Read the model definition and answer for the solid it produces. Units are mm, in the model's axes. A direction names the side the tool comes from. Coordinates: 2 decimals unless noted, no trailing zeros. Order: outer loops, then holes, each group sorted by start corner. A loop starts at its lowest first (then second) coordinate and runs counter-clockwise, first axis right, second up. Notation, with made-up numbers: M 34,-38.75 L 59,-38.75 A17 cw 59,-14.75 Z; hole C 16.5,36.25 d9. An arc over 180 degrees is marked long. One line per question, with ' | ' between items. Start each with the question number.
1) A tool of negligible diameter and unlimited length cuts with its end or side. For faces 1 (the face through (7, -7, 0)), 2 (the face through (-7.559, -5.796, 36.51)), from which of +Z, -Z, +X, -X, +Y, -Y can it reach the whole face along a straight path? Write none if from no direction.
2) Consider probe 1 along X at (y, z) = (7, 51.5); probe 2 along X at (y, z) = (8.5, 41); probe 3 along Y at (x, z) = (2, 38.5). Determine where each line is inside the solid, lowest interval first.
3) Find section A-A, the plane z = 38. Count the separate pieces of the cut face and the enclosed holes in it, plus the area to 3 significant figures.
4) The mould has two halves that part along Y. Classify faces 3 (the face through (-6.883, -30.995, 35.496)), 4 (the face through (-2, 8, 72)), 5 (the face through (-1.72, -7.75, 35.5)): +Y half, -Y half, draft (parallel to the pull), parting line (faces both ways), or undercut.
5) Find section D-D, the plane y = -19.5. Write down the section's boundary in (x, z), plus the area to 3 significant figures.
6) Given P1, Ø3, axis at y = 2, z = 23, coming from the +X side; P2, Ø1.5, axis at y = 23, z = 64.5, coming from the +X side; P3, Ø10, axis at x = -6, z = 23.5, coming from the -Y side, each flat-ended and moving along its own axis, determine where each tip first touches the part or whether it passes through.
from build123d import *

# Parameters (mm, degrees)
CROQUIS1_R              = 31.75
CROQUIS1_R_2            = 7.9375
SALIENTE_EXTRUIR1_DEPTH = 2
CROQUIS2_R              = 31.75
CROQUIS2_R_2            = 29.75
SALIENTE_EXTRUIR2_DEPTH = 70
CROQUIS3_R              = 9.525
CROQUIS3_R_2            = 7.9375
SALIENTE_EXTRUIR3_DEPTH = 70


with BuildPart() as part:
    # Croquis1 → Saliente-Extruir1 (new body)
    with BuildSketch(Plane.XY):
        Circle(CROQUIS1_R)
        Circle(CROQUIS1_R_2, mode=Mode.SUBTRACT)
    extrude(amount=SALIENTE_EXTRUIR1_DEPTH)

    # Croquis2 → Saliente-Extruir2 (add)
    with BuildSketch(Plane.XY.offset(2)):
        Circle(CROQUIS2_R)
        Circle(CROQUIS2_R_2, mode=Mode.SUBTRACT)
    extrude(amount=SALIENTE_EXTRUIR2_DEPTH)

    # Croquis3 → Saliente-Extruir3 (add)
    with BuildSketch(Plane.XY.offset(2)):
        Circle(CROQUIS3_R)
        Circle(CROQUIS3_R_2, mode=Mode.SUBTRACT)
    extrude(amount=SALIENTE_EXTRUIR3_DEPTH)


solid = part.part
Report:
1) face 1: -Z, +X, -X, +Y, -Y | face 2: +Z
2) probe 1: x = -30.97 to -28.91, -6.46 to -3.74, 3.74 to 6.46, 28.91 to 30.97 | probe 2: x = -30.59 to -28.51, -4.3 to 4.3, 28.51 to 30.59 | probe 3: y = -31.69 to -29.68, -9.31 to -7.68, 7.68 to 9.31, 29.68 to 31.69
3) separate pieces: 2 | enclosed holes: 2 | area: 474 mm^2
4) face 3: parting line | face 4: draft | face 5: undercut
5) outline: M -25.06,0 L 25.06,0 L 25.06,72 L 22.47,72 L 22.47,2 L -22.47,2 L -22.47,72 L -25.06,72 Z | area: 463 mm^2
6) P1: stops at x = 31.75 | P2: stops at x = 22.65 | P3: stops at y = -31.73
